Can you work these out from the model? Positions are in its coordinate system, mm. A direction names the side the tool comes from. Round coordinates to 2 decimals unless told otherwise and drop trailing zeros. Loops run counter-clockwise (first coordinate to the right, second up) from the corner with the lowest first, then second, coordinate; pieces in that order, holes last. Notation, with made-up numbers: (3.25, 33) -> (38.25, 33) arc R21 ccw to (38.25, 44) -> close; hole circle Ø6 at (48.25, 83.25). An arc over 180 degrees is marked (long way). Use a Markdown table: item, result.
from build123d import *

# Parameters (mm, degrees)
F0_R     = 30
F1_DEPTH = 30
F2_DEPTH = 20
F3_DEPTH = 20


with BuildPart() as f1:
    # F0 (on Front) → F1 (new body)
    with BuildSketch(Plane.XZ):
        Circle(F0_R)
    extrude(amount=F1_DEPTH)

    # F0 (on Front) → F2 (join)
    with BuildSketch(Plane.XZ):
        with BuildLine():
            ThreePointArc((-6.23154, 99.805651), (-68.47206, -72.880567), (100, 0))
            ThreePointArc((100, 0), (75.397007, 65.690877), (13.694172, 99.057911))
            ThreePointArc((13.694172, 99.057911), (3.75, 99.929663), (-6.23154, 99.805651))
        make_face()
        Circle(F0_R, mode=Mode.SUBTRACT)
    extrude(amount=F2_DEPTH)

    # F0 (on Front) → F3 (join)
    with BuildSketch(Plane.XZ):
        with BuildLine():
            ThreePointArc((-6.23154, 99.805651), (3.75, 99.929663), (13.694172, 99.057911))
            Line((13.694172, 99.057911), (8.99367, 119.6625))
            Line((8.99367, 119.6625), (0, 120))
            Line((0, 120), (-6.23154, 99.805651))
        make_face()
    extrude(amount=F3_DEPTH)


solid = f1.part
1. I want a section at A-A (y = -13.25). Please give me the cut outline in (x, z), plus the area to 3 significant figures.
Answer sheet:
| item | result |
|---|---|
| outline | (-6.23, 99.81) arc R100 ccw (long way) to (13.69, 99.06) -> (8.99, 119.66) -> (0, 120) -> close |
| area | 31,700 mm² |
2. I want a section at B-B (z = 80). Please give me the cut outline in (x, y).
Answer sheet:
| item | result |
|---|---|
| outline | (-60, -20) -> (60, -20) -> (60, 0) -> (-60, 0) -> close |
3. Will these pins go through, and if not, where does the flat tip stop? pin 1 Ø12 at (x, y) = (35.5, -12.5) entering from -Z; pin 2 Ø8 at (x, z) = (-70, 30.5) entering from -Y; pin 3 Ø8 at (x, z) = (-44, 84) entering from +Y; pin 4 Ø4 at (x, y) = (-23.5, -4.5) entering from +Z.
Answer sheet:
| item | result |
|---|---|
| pin 1 | stops at z = -95.55 |
| pin 2 | stops at y = -20 |
| pin 3 | stops at y = 0 |
| pin 4 | stops at z = 97.66 |
4. I want a section at C-C (x = 60). Please give me the cut outline in (y, z), plus the area to 3 significant figures.
Answer sheet:
| item | result |
|---|---|
| outline | (-20, -80) -> (0, -80) -> (0, 80) -> (-20, 80) -> close |
| area | 3,200 mm² |
5. I need wall thicknesses on line 1 (Y direction, x = -28, z = -63); line 2 (X direction, y = -11.75, z = 86.5); line 3 (Z direction, x = -50, y = -5). Which ranges of each line are inside material? Lowest first, please.
Answer sheet:
| item | result |
|---|---|
| line 1 | y = -20 to 0 |
| line 2 | x = -50.18 to 50.18 |
| line 3 | z = -86.6 to 86.6 |
6. Which directions (+Z, -Z, +X, -X, +Y, -Y) give clear straight access to the entire face, cutting with the end or side of a thin tool? Please do faces 1 (the cylindrical face through (-29.97, -24.93, 1.32)), 2 (the flat face through (0, -30, 0)).
Answer sheet:
| item | result |
|---|---|
| face 1 | -Y |
| face 2 | +Z, -Z, +X, -X, -Y |
7. I want a section at D-D (y = -26.5). Please give me the cut outline in (x, z), plus the area to 3 significant figures.
Answer sheet:
| item | result |
|---|---|
| outline | circle Ø60 at (0, 0) |
| area | 2,830 mm² |
